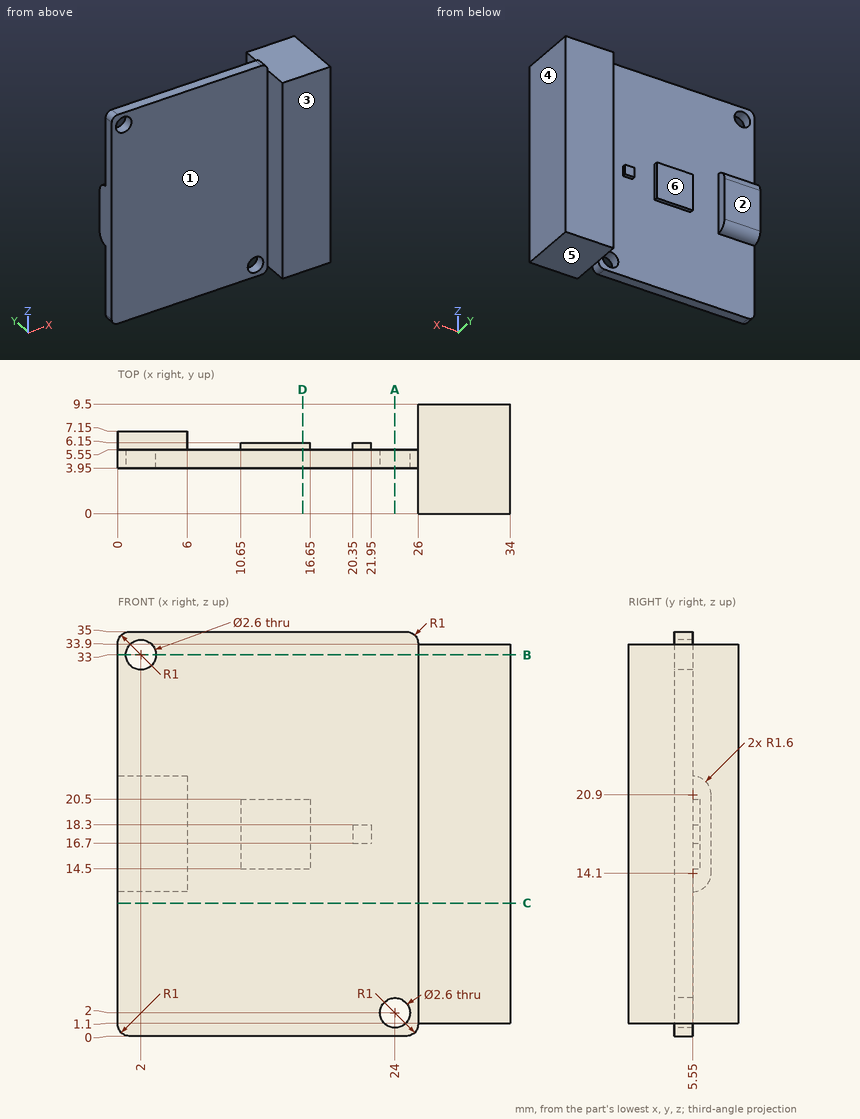
Source: three-view drawing plus pictorial views. Frame: mm from the lowest corner of the part. A direction names the side the tool comes from. Round coordinates to 2 decimals unless told otherwise and drop trailing zeros. Loops run counter-clockwise (first coordinate to the right, second up) from the corner with the lowest first, then second, coordinate; pieces in that order, holes last. Notation, with made-up numbers: M 89.5,77 L 104.5,77 A22 ccw 104.5,96 Z; hole C 18,69.25 d5. An arc over 180 degrees is marked long. Answer as CSV lines item,"result". Start each with the question number.
(1) Section A-A, the plane x = 24. Output: boundary loops of the cut face in (y, z).
(2) Section C-C, the plane z = 11.5. Output: boundary loops of the cut face in (x, y), plus the area to 3 significant figures.
(3) Reachability of the marked faces 1, 2 and 3 from +Z, -Z, +X, -X, +Y, -Y: full face, straight path, thin tool, end or side. Return the list, or none.
(4) Draft query along X for the marked faces 4, 5 and 6. Return one class per face: released by +X, released by -X, zero draft, split by the parting line, or undercut.
(5) Line query: line 1 (Z direction, x = 2, y = 4.95); line 2 (Z direction, x = 24, y = 4.45); line 3 (X direction, y = 4, z = 33). Output: solid intervals per line, ascending. Write a range as [from, to].
(6) First-contact query: pin 1 (1.2 mm diameter, centred on y = 2, z = 21, fed in from -X); pin 2 (3.5 mm diameter, centred on x = 24, z = 2, fed in from +Y); pin 3 (0.8 mm diameter, centred on x = 21.5, z = 17, fed in from +Y). Flat tips, straight axial feed; report the tip coordinate or a pass-through.
(7) Section B-B, the plane z = 33. Output: boundary loops of the cut face in (x, y).
(8) Section D-D, the plane x = 16. Output: boundary loops of the cut face in (y, z), plus the area to 3 significant figures.
Values found:
1,outline,"M 3.95,0 L 5.55,0 L 5.55,0.7 L 3.95,0.7 Z; M 3.95,3.3 L 5.55,3.3 L 5.55,35 L 3.95,35 Z"
2,outline,"M 0,3.95 L 26,3.95 L 26,0 L 34,0 L 34,9.5 L 26,9.5 L 26,5.55 L 0,5.55 Z"
2,area,"118 mm²"
3,face 1,"+Z, -Z, -X, -Y"
3,face 2,"+Z, -Z, -X, +Y"
3,face 3,"+Z, -Z, +X, -X, -Y"
4,face 4,"released by +X"
4,face 5,"zero draft"
4,face 6,"undercut"
5,line 1,"z = [0, 31.7], [34.3, 35]"
5,line 2,"z = [0, 0.7], [3.3, 35]"
5,line 3,"x = [0, 0.7], [3.3, 34]"
6,pin 1,"stops at x = 26"
6,pin 2,"stops at y = 5.55"
6,pin 3,"stops at y = 6.15"
7,outline,"M 0,3.95 L 0.7,3.95 L 0.7,5.55 L 0,5.55 Z; M 3.3,3.95 L 26,3.95 L 26,0 L 34,0 L 34,9.5 L 26,9.5 L 26,5.55 L 3.3,5.55 Z"
8,outline,"M 3.95,0 L 5.55,0 L 5.55,14.5 L 6.15,14.5 L 6.15,20.5 L 5.55,20.5 L 5.55,35 L 3.95,35 Z"
8,area,"59.6 mm²"
